Could you check a few things on this model? Use its own coordinates, in mm. A direction names the side the tool comes from. Round coordinates to 2 decimals unless told otherwise and drop trailing zeros. Order: outer loops, then holes, each group sorted by start corner. A loop starts at its lowest first (then second) coordinate and runs counter-clockwise, first axis right, second up. Notation, with made-up numbers: (-38, 89.5) -> (-14, 89.5) arc R29 cw to (-14, 128.5) -> close; hole circle Ø10 at (14, 17.25). An arc over 180 degrees is marked (long way). One line per question, with ' | ' between items.
```python
from build123d import *

# Parameters (mm, degrees)
BOX085056_W     = 4
BOX085056_H     = 58
BOX085056_DEPTH = 4
BOX085057_W     = 4
BOX085057_H     = 4
BOX085057_DEPTH = 20
BOX085058_W     = 4
BOX085058_H     = 4
BOX085058_DEPTH = 20
BOX085059_W     = 4
BOX085059_H     = 4
BOX085059_DEPTH = 20
BOX085060_W     = 4
BOX085060_H     = 4
BOX085060_DEPTH = 20
BOX085061_W     = 4
BOX085061_H     = 4
BOX085061_DEPTH = 20
BOX085062_W     = 4
BOX085062_H     = 4
BOX085062_DEPTH = 20
BOX085063_W     = 4
BOX085063_H     = 4
BOX085063_DEPTH = 20
BOX085064_W     = 4
BOX085064_H     = 4
BOX085064_DEPTH = 20
BOX085065_W     = 38
BOX085065_H     = 4
BOX085065_DEPTH = 4
BOX085066_W     = 38
BOX085066_H     = 4
BOX085066_DEPTH = 4
BOX085067_W     = 4
BOX085067_H     = 4
BOX085067_DEPTH = 20
BOX085068_W     = 4
BOX085068_H     = 4
BOX085068_DEPTH = 20
BOX085069_W     = 4
BOX085069_H     = 4
BOX085069_DEPTH = 20
BOX085070_W     = 4
BOX085070_H     = 4
BOX085070_DEPTH = 20
BOX085055_W     = 4
BOX085055_H     = 58
BOX085055_DEPTH = 4


with BuildPart() as cube142:
    # Box085056 → Box085056 (new body)
    with BuildSketch(Plane(origin=(107, 2, 22), x_dir=(1, 0, 0), z_dir=(0, 0, 1))):
        with Locations((2, 29)):
            Rectangle(BOX085056_W, BOX085056_H)
    extrude(amount=BOX085056_DEPTH)


with BuildPart() as cube143:
    # Box085057 → Box085057 (new body)
    with BuildSketch(Plane(origin=(65, 38, 2), x_dir=(1, 0, 0), z_dir=(0, 0, 1))):
        with Locations((2, 2)):
            Rectangle(BOX085057_W, BOX085057_H)
    extrude(amount=BOX085057_DEPTH)


with BuildPart() as cube144:
    # Box085058 → Box085058 (new body)
    with BuildSketch(Plane(origin=(65, 2, 2), x_dir=(1, 0, 0), z_dir=(0, 0, 1))):
        with Locations((2, 2)):
            Rectangle(BOX085058_W, BOX085058_H)
    extrude(amount=BOX085058_DEPTH)


with BuildPart() as cube145:
    # Box085059 → Box085059 (new body)
    with BuildSketch(Plane(origin=(65, 56, 2), x_dir=(1, 0, 0), z_dir=(0, 0, 1))):
        with Locations((2, 2)):
            Rectangle(BOX085059_W, BOX085059_H)
    extrude(amount=BOX085059_DEPTH)


with BuildPart() as cube146:
    # Box085060 → Box085060 (new body)
    with BuildSketch(Plane(origin=(107, 38, 2), x_dir=(1, 0, 0), z_dir=(0, 0, 1))):
        with Locations((2, 2)):
            Rectangle(BOX085060_W, BOX085060_H)
    extrude(amount=BOX085060_DEPTH)


with BuildPart() as cube147:
    # Box085061 → Box085061 (new body)
    with BuildSketch(Plane(origin=(107, 2, 2), x_dir=(1, 0, 0), z_dir=(0, 0, 1))):
        with Locations((2, 2)):
            Rectangle(BOX085061_W, BOX085061_H)
    extrude(amount=BOX085061_DEPTH)


with BuildPart() as cube148:
    # Box085062 → Box085062 (new body)
    with BuildSketch(Plane(origin=(107, 56, 2), x_dir=(1, 0, 0), z_dir=(0, 0, 1))):
        with Locations((2, 2)):
            Rectangle(BOX085062_W, BOX085062_H)
    extrude(amount=BOX085062_DEPTH)


with BuildPart() as cube149:
    # Box085063 → Box085063 (new body)
    with BuildSketch(Plane(origin=(65, 20, 2), x_dir=(1, 0, 0), z_dir=(0, 0, 1))):
        with Locations((2, 2)):
            Rectangle(BOX085063_W, BOX085063_H)
    extrude(amount=BOX085063_DEPTH)


with BuildPart() as cube150:
    # Box085064 → Box085064 (new body)
    with BuildSketch(Plane(origin=(107, 20, 2), x_dir=(1, 0, 0), z_dir=(0, 0, 1))):
        with Locations((2, 2)):
            Rectangle(BOX085064_W, BOX085064_H)
    extrude(amount=BOX085064_DEPTH)


with BuildPart() as cube151:
    # Box085065 → Box085065 (new body)
    with BuildSketch(Plane(origin=(69, 20, 22), x_dir=(1, 0, 0), z_dir=(0, 0, 1))):
        with Locations((19, 2)):
            Rectangle(BOX085065_W, BOX085065_H)
    extrude(amount=BOX085065_DEPTH)


with BuildPart() as cube152:
    # Box085066 → Box085066 (new body)
    with BuildSketch(Plane(origin=(69, 38, 22), x_dir=(1, 0, 0), z_dir=(0, 0, 1))):
        with Locations((19, 2)):
            Rectangle(BOX085066_W, BOX085066_H)
    extrude(amount=BOX085066_DEPTH)


with BuildPart() as cube153:
    # Box085067 → Box085067 (new body)
    with BuildSketch(Plane(origin=(79, 20, 2), x_dir=(1, 0, 0), z_dir=(0, 0, 1))):
        with Locations((2, 2)):
            Rectangle(BOX085067_W, BOX085067_H)
    extrude(amount=BOX085067_DEPTH)


with BuildPart() as cube154:
    # Box085068 → Box085068 (new body)
    with BuildSketch(Plane(origin=(93, 20, 2), x_dir=(1, 0, 0), z_dir=(0, 0, 1))):
        with Locations((2, 2)):
            Rectangle(BOX085068_W, BOX085068_H)
    extrude(amount=BOX085068_DEPTH)


with BuildPart() as cube155:
    # Box085069 → Box085069 (new body)
    with BuildSketch(Plane(origin=(79, 38, 2), x_dir=(1, 0, 0), z_dir=(0, 0, 1))):
        with Locations((2, 2)):
            Rectangle(BOX085069_W, BOX085069_H)
    extrude(amount=BOX085069_DEPTH)


with BuildPart() as cube156:
    # Box085070 → Box085070 (new body)
    with BuildSketch(Plane(origin=(93, 38, 2), x_dir=(1, 0, 0), z_dir=(0, 0, 1))):
        with Locations((2, 2)):
            Rectangle(BOX085070_W, BOX085070_H)
    extrude(amount=BOX085070_DEPTH)


with BuildPart() as drawer_rails:
    # Box085055 → Box085055 (new body)
    with BuildSketch(Plane(origin=(65, 2, 22), x_dir=(1, 0, 0), z_dir=(0, 0, 1))):
        with Locations((2, 29)):
            Rectangle(BOX085055_W, BOX085055_H)
    extrude(amount=BOX085055_DEPTH)

    # Fusion004008002002002001007002002018: union Cube142, Cube143, Cube144, Cube145, Cube146, Cube147, Cube148, Cube149, Cube150, Cube151, Cube152, Cube153, Cube154, Cube155, Cube156
    add(cube142.part)
    add(cube143.part)
    add(cube144.part)
    add(cube145.part)
    add(cube146.part)
    add(cube147.part)
    add(cube148.part)
    add(cube149.part)
    add(cube150.part)
    add(cube151.part)
    add(cube152.part)
    add(cube153.part)
    add(cube154.part)
    add(cube155.part)
    add(cube156.part)


solid = drawer_rails.part
```
1. If we mould it in two halves opening along Y, with no side actions, what happens to faces 4 (the face through (67, 2, 14)), 5 (the face through (97, 40, 12)), 6 (the face through (109, 6, 12)), 7 (the face through (67, 38, 12))? For each: pulls with the +Y half, pulls with the -Y half, needs draft (parallel to the pull), parting line crosses it, or undercut.
From the geometry:
face 4: pulls with the -Y half | face 5: needs draft | face 6: undercut | face 7: undercut
2. I want a section at B-B on z = 23.75. List the corners of the cut face in (x, y) for me.
From the geometry:
outline: (65, 2) -> (69, 2) -> (69, 20) -> (107, 20) -> (107, 2) -> (111, 2) -> (111, 60) -> (107, 60) -> (107, 42) -> (69, 42) -> (69, 60) -> (65, 60) -> close; hole (69, 24) -> (107, 24) -> (107, 38) -> (69, 38) -> close
3. On a 3-axis mill with a long thin cutter (end or side, diameter ignored), from which of +Z, -Z, +X, -X, +Y, -Y can I reach the whole of each face in a straight line? I mean faces 1 (the face through (69, 5.6, 16.6)), 2 (the face through (93, 22, 12)), 3 (the face through (109, 49, 22)). Say none if no direction works.
From the geometry:
face 1: +Z, -Z, -Y | face 2: -Z, +Y, -Y | face 3: -Z, +X, -X
4. I want a section at C-C on y = 34. List the corners of the cut face in (x, z) for me, and give its area (3 significant figures).
From the geometry:
outline: (65, 22) -> (69, 22) -> (69, 26) -> (65, 26) -> close; (107, 22) -> (111, 22) -> (111, 26) -> (107, 26) -> close | area: 32.0 mm²
5. I want a section at A-A on x = 87. List the corners of the cut face in (y, z) for me.
From the geometry:
outline: (20, 22) -> (24, 22) -> (24, 26) -> (20, 26) -> close; (38, 22) -> (42, 22) -> (42, 26) -> (38, 26) -> close
6. I need wall thicknesses on probe 1 along X at (y, z) = (41.5, 18.25); probe 2 along Y at (x, z) = (108.5, 12.25); probe 3 along Y at (x, z) = (74.5, 24.75). Which ranges of each line are inside material? Lowest first, please.
From the geometry:
probe 1: x = 65 to 69, 79 to 83, 93 to 97, 107 to 111 | probe 2: y = 2 to 6, 20 to 24, 38 to 42, 56 to 60 | probe 3: y = 20 to 24, 38 to 42
7. I want a section at D-D on y = 23. List the corners of the cut face in (x, z) for me.
From the geometry:
outline: (65, 2) -> (69, 2) -> (69, 22) -> (79, 22) -> (79, 2) -> (83, 2) -> (83, 22) -> (93, 22) -> (93, 2) -> (97, 2) -> (97, 22) -> (107, 22) -> (107, 2) -> (111, 2) -> (111, 26) -> (65, 26) -> close
8. I'm going to push flat-ended pins straight in: pin 1 (5 mm diameter, centred on x = 72, z = 10.5, fed in from -Y); pin 2 (4.5 mm diameter, centred on x = 99.5, y = 39.5, fed in from -Z); pin 3 (6 mm diameter, centred on x = 97, z = 12.5, fed in from -Y). Where does each tip first touch, or does it pass through?
From the geometry:
pin 1: passes through | pin 2: stops at z = 22 | pin 3: stops at y = 20
